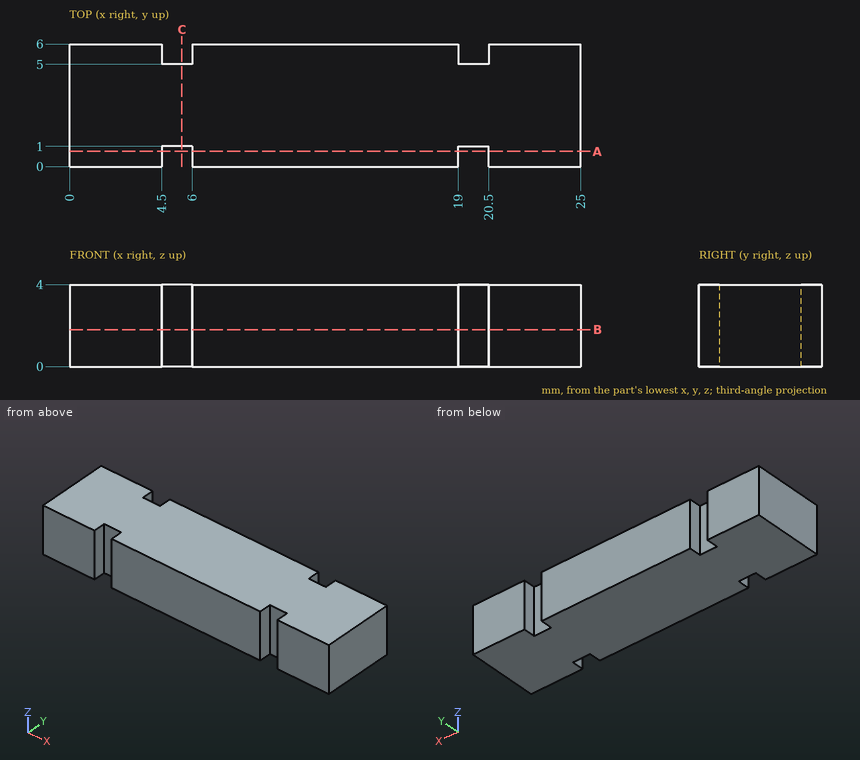
Geometry check sheet. Reference: drawing and pictorial views, mm from the part's lowest x, y, z. Coordinates: 2 decimals unless noted, no trailing zeros. Order: outer loops, then holes, each group sorted by start corner. A loop starts at its lowest first (then second) coordinate and runs counter-clockwise, first axis right, second up. Notation, with made-up numbers: (-16, 12) -> (24, 12) arc R30 cw to (24, 51) -> close; hole circle Ø2 at (-14, 54). An arc over 180 degrees is marked (long way). Use CSV: the item, a comma, the result in double quotes. Start each with the question number.
Q1. Section check B-B, the plane z = 1.8. Record the cut outline in (x, y), and give its area (3 significant figures).
Q2. Section check C-C, the plane x = 5.5. Record the cut outline in (y, z).
Q3. Section check A-A, the plane y = 0.75. Record the cut outline in (x, z), and give its area (3 significant figures).
Q4. Thickness scan on line 1 along X through (y, z) = (5.05, 1.45); line 2 along Y through (x, z) = (5.5, 2). Record the ranges inside material, lowest first.
Returned:
1,outline,"(0, 0) -> (4.5, 0) -> (4.5, 1) -> (6, 1) -> (6, 0) -> (19, 0) -> (19, 1) -> (20.5, 1) -> (20.5, 0) -> (25, 0) -> (25, 6) -> (20.5, 6) -> (20.5, 5) -> (19, 5) -> (19, 6) -> (6, 6) -> (6, 5) -> (4.5, 5) -> (4.5, 6) -> (0, 6) -> close"
1,area,"144 mm^2"
2,outline,"(1, 0) -> (5, 0) -> (5, 4) -> (1, 4) -> close"
3,outline,"(0, 0) -> (4.5, 0) -> (4.5, 4) -> (0, 4) -> close; (6, 0) -> (19, 0) -> (19, 4) -> (6, 4) -> close; (20.5, 0) -> (25, 0) -> (25, 4) -> (20.5, 4) -> close"
3,area,"88.0 mm^2"
4,line 1,"x = 0 to 4.5, 6 to 19, 20.5 to 25"
4,line 2,"y = 1 to 5"
